Could you check a few things on this model? Use its own coordinates, in mm. A direction names the side the tool comes from. Give positions to 0.01 mm unless a question says otherwise; leave off trailing zeros. Loops run counter-clockwise (first coordinate to the right, second up) from the corner with the lowest first, then second, coordinate; pieces in that order, holes last. Notation, with made-up numbers: (57, 54) - (68, 54) arc R25 cw to (68, 80) - close; hole circle Ø2 at (81, -29). An arc over 180 degrees is marked (long way). Use CSV: the item, a comma, the result in double quotes.
Autodesk Fusion 360 part; units mm, degrees
sketch "Sketch1" plane through (0, 0, 0) normal (0, 1, 0) x (1, 0, 0)
  circle A0 centre (0, 0) radius 8
  circle A1 centre (0, 0) radius 12.5
  line L0 (0, 0) -> (12.5, 0)
  line L1 (0, 0) -> (0, -12.5)
  dimension "d1" = 16
  dimension "d2" = 25
extrude "Extrude1" add sketch "Sketch1" along normal blind 20 contours A0 A1 L0 L1 picked at (-5.2365, -9.6417)
fillet "Fillet1" radius 2 2 edges at (8, 10, 0) (0, 10, 8)
fillet "Fillet2" radius 0.5 2 edges at (0, 10, 12.5) (12.5, 10, 0)
1) We'd pull the mould along Z, two halves only. Please class faces 4 (the cylindrical face through (-5.825, 9.86, -5.484)), 5 (the cylindrical face through (8.52, 10.14, -0.46)), 6 (the flat face through (-6, 0, -6)): +Z half, -Z half, draft (parallel to the pull), parting line (faces both ways), or undercut.
Answer below:
face 4,"undercut"
face 5,"+Z half"
face 6,"draft"
2) Suppose I cut it at B-B (x = -7). Please give me the cut outline in (y, z).
Answer below:
outline,"(0, -10.36) - (20, -10.36) - (20, -3.87) - (0, -3.87) - close; (0, 3.87) - (20, 3.87) - (20, 10.36) - (0, 10.36) - close"
3) Suppose I cut it at C-C (y = 11.25). Please give me the cut outline in (x, z), plus the area to 3 significant figures.
Answer below:
outline,"(-1.6, 7.84) arc R2 ccw to (0, 9.8) - (0, 11.99) arc R0.5 ccw to (-0.52, 12.49) arc R12.5 ccw (long way) to (12.49, -0.52) arc R0.5 ccw to (11.99, 0) - (9.8, 0) arc R2 ccw to (7.84, -1.6) arc R8 cw (long way) to start"
area,"216 mm2"
4) I need wall thicknesses on line 1 along Z through (x, y) = (-1.25, 5); line 2 along Z through (x, y) = (-3.75, 13.5); line 3 along X through (y, z) = (8, -3.5). Which ranges of each line are inside material? Lowest first, please.
Answer below:
line 1,"z = -12.44 to -7.9, 7.94 to 12.44"
line 2,"z = -11.92 to -7.07, 7.07 to 11.92"
line 3,"x = -12 to -7.19, 7.19 to 12"
5) Suppose I cut it at D-D (x = 10.75). Please give me the cut outline in (y, z).
Answer below:
outline,"(0, -6.38) - (20, -6.38) - (20, 0) - (0, 0) - close"
6) Which directions (+Z, -Z, +X, -X, +Y, -Y) give clear straight access to the entire face, cutting with the end or side of a thin tool? Please do faces 1 (the cylindrical face through (-0.439, 10.14, 8.548)), 2 (the flat face through (-6, 20, -6)), 3 (the flat face through (0, 10, 11)).
Answer below:
face 1,"+X, +Y, -Y"
face 2,"+Z, -Z, +X, -X, +Y"
face 3,"+Z, +X, +Y, -Y"
7) I'm going to push flat-ended pins straight in: P1, Ø10, axis at x = 6, y = 18, coming from the -Z side; P2, Ø1, axis at y = 12.5, z = 1, coming from the -X side; P3, Ø6, axis at x = 7.5, y = 8.5, coming from the -Z side. Where does each tip first touch, or does it pass through?
Answer below:
P1,"stops at z = -12.46"
P2,"stops at x = -12.49"
P3,"stops at z = -11.66"
8) Suppose I cut it at A-A (z = -7.25). Please give me the cut outline in (x, y).
Answer below:
outline,"(-10.18, 0) - (-3.38, 0) - (-3.38, 20) - (-10.18, 20) - close; (3.38, 0) - (10.18, 0) - (10.18, 20) - (3.38, 20) - close"
